Verification items for the finished model (mm, model axes). A direction names the side the tool comes from. Round coordinates to 2 decimals unless told otherwise and drop trailing zeros. Write each loop counter-clockwise with the first axis right and the second up, starting at its lowest first coordinate (ties: lowest second). Pieces come first, ordered by that corner, then holes. Notation, with made-up numbers: (21, 30) - (79, 30) arc R21 ccw to (79, 55) - close; hole circle Ø9 at (-10.5, -7). An arc over 180 degrees is marked (long way). Answer as a JSON object with one key per item and string values.
Autodesk Fusion 360 part; units mm, degrees
sketch "Sketch1" plane through (0, 0, 0) normal (0, 0, 1) x (1, 0, 0)
  line L0 (0, 0) -> (6.5, 0)
  line L1 (6.5, 0) -> (6.5, 6.5)
  line L2 (6.5, 6.5) -> (0, 6.5)
  line L3 (0, 6.5) -> (0, 0)
  line L4 (0, 3.25) -> (6.5, 3.25) construction
  line L5 (3.25, 6.5) -> (3.25, 0) construction
  circle A0 centre (3.25, 3.25) radius 1.75
  line L6 (-1.4, 7.9) -> (-1.4, -1.4)
  line L7 (-1.4, -1.4) -> (7.9, -1.4)
  line L8 (7.9, -1.4) -> (7.9, 7.9)
  line L9 (7.9, 7.9) -> (-1.4, 7.9)
  line L10 (-3, 9.5) -> (-3, -3)
  line L11 (-3, -3) -> (9.5, -3)
  line L12 (9.5, -3) -> (9.5, 9.5)
  line L13 (9.5, 9.5) -> (-3, 9.5)
  dimension "d1" = 6.5
  dimension "d2" = 6.5
  dimension "d3" = 3.5
  dimension "d4" = 1.4
  dimension "d5" = 3
extrude "Extrude1" add sketch "Sketch1" along normal blind 7 contours L6 L7 L8 L9
extrude "Extrude2" add sketch "Sketch1" along normal blind 1.5 from surface at 1.5 contours L10 L11 L12 L13
extrude "Extrude3" add sketch "Sketch1" along normal blind 3.5 from surface at 3.5 contours L0 L1 L2 L3 | A0
extrude "Extrude4" cut sketch "Sketch1" along normal blind 4 contours A0
1. Go/stop test with flat-tipped pins: pin 1 (1.5 mm diameter, centred on y = 2, z = 5, fed in from +X); pin 2 (0.8 mm diameter, centred on x = 4, z = 0.5, fed in from -Y); pin 3 (4 mm diameter, centred on x = 4, y = 4, fed in from -Z). Record where each tip stops, or that it passes through.
Completed:
{"pin 1": "stops at x = 7.9", "pin 2": "stops at y = -1.4", "pin 3": "stops at z = 3.5"}
2. Material ranges on probe 1 along Y at (x, z) = (3.25, 3.95); probe 2 along X at (y, z) = (6, 1.75), recorded low to high. Write a range as from..to.
Completed:
{"probe 1": "y = -1.4..1.5, 5..7.9", "probe 2": "x = -3..0, 6.5..9.5"}
3. Cross-section at C-C (x = 5.5). Record the boundary of the cut face in (y, z).
Completed:
{"outline": "(-3, 1.5) - (-1.4, 1.5) - (-1.4, 0) - (0, 0) - (0, 3.5) - (6.5, 3.5) - (6.5, 0) - (7.9, 0) - (7.9, 1.5) - (9.5, 1.5) - (9.5, 3) - (7.9, 3) - (7.9, 7) - (-1.4, 7) - (-1.4, 3) - (-3, 3) - close"}
4. Cross-section at A-A (z = 2.5). Record the boundary of the cut face in (x, y), plus the area to 3 significant figures.
Completed:
{"outline": "(-3, -3) - (9.5, -3) - (9.5, 9.5) - (-3, 9.5) - close; hole (0, 0) - (6.5, 0) - (6.5, 6.5) - (0, 6.5) - close", "area": "114 mm^2"}
5. Mould release check, pull along Y, two halves, no side actions. Record for faces 1 (the face through (3, -1.4, 1)), 2 (the face through (0, 3, 2)), 3 (the face through (-3, 3, 2)): released by +Y, released by -Y, zero draft, split by the parting line, or undercut.
Completed:
{"face 1": "released by -Y", "face 2": "undercut", "face 3": "zero draft"}
6. Access from +Z, -Z, +X, -X, +Y, -Y to the whole of each face (thin tool, end or side, straight path). Record for faces 4 (the face through (7.9, 3, 1)), 5 (the face through (6.5, 3, 2)), 6 (the face through (3, 7.9, 5)), 7 (the face through (3, -1.4, 5)).
Completed:
{"face 4": "-Z, +X, +Y, -Y", "face 5": "-Z", "face 6": "+Z, +X, -X, +Y", "face 7": "+Z, +X, -X, -Y"}
7. Cross-section at B-B (y = 3.25). Record the boundary of the cut face in (x, z).
Completed:
{"outline": "(-3, 1.5) - (-1.4, 1.5) - (-1.4, 0) - (0, 0) - (0, 3.5) - (1.5, 3.5) - (1.5, 4) - (5, 4) - (5, 3.5) - (6.5, 3.5) - (6.5, 0) - (7.9, 0) - (7.9, 1.5) - (9.5, 1.5) - (9.5, 3) - (7.9, 3) - (7.9, 7) - (-1.4, 7) - (-1.4, 3) - (-3, 3) - close"}
